from build123d import *

# Parameters (mm, degrees)
SKETCH1_R           = 13.5
BOSS_EXTRUDE1_DEPTH = 60
CUT_EXTRUDE1_START  = -30
SKETCH2_R           = 13.5
SKETCH2_R_2         = 12
CUT_EXTRUDE1_DEPTH  = 30
SKETCH3_R           = 2
BOSS_EXTRUDE2_DEPTH = 7
SKETCH4_W           = 23.8117618
SKETCH4_H           = 3
BOSS_EXTRUDE3_DEPTH = 2


with BuildPart() as part:
    # Sketch1 → Boss-Extrude1 (new body)
    with BuildSketch(Plane.XY):
        Circle(SKETCH1_R)
    extrude(amount=BOSS_EXTRUDE1_DEPTH)

    # Sketch2 → Cut-Extrude1 (cut)
    with BuildSketch(Plane.XY.offset(60).offset(CUT_EXTRUDE1_START)):
        Circle(SKETCH2_R)
        Circle(SKETCH2_R_2, mode=Mode.SUBTRACT)
    extrude(amount=CUT_EXTRUDE1_DEPTH, mode=Mode.SUBTRACT)

    # Sketch3 → Boss-Extrude2 (add)
    with BuildSketch(Plane(origin=(0, 0, 0), x_dir=(-1, 0, 0), z_dir=(0, 0, -1))):
        Circle(SKETCH3_R)
        with Locations(Location((-8, 0, 0), (0, 0, 180))):
            Circle(SKETCH3_R)
    extrude(amount=BOSS_EXTRUDE2_DEPTH)

    # Sketch4 → Boss-Extrude3 (add)
    with BuildSketch(Plane.XY.offset(60)):
        Rectangle(SKETCH4_W, SKETCH4_H)
    extrude(amount=BOSS_EXTRUDE3_DEPTH)


solid = part.part
CAD build for the part. Positions are in the model's coordinates, mm. A direction names the side the tool comes from. Coordinates: 2 decimals unless noted, no trailing zeros. Write each loop counter-clockwise with the first axis right and the second up, starting at its lowest first coordinate (ties: lowest second). Pieces come first, ordered by that corner, then holes. Notation, with made-up numbers: M 52,84 L 107,84 A28 ccw 107,107 Z; hole C 76.25,-4.5 d8. An arc over 180 degrees is marked long. Return JSON: item names as keys, results as strings.
Item 1: Drop flat-ended pins along their axis: pin 1 Ø1.5 at (x, y) = (6.5, 3) entering from +Z; pin 2 Ø1.6 at (y, z) = (-0.5, 61) entering from -X; pin 3 Ø5 at (x, z) = (-10.5, 49.5) entering from +Y. Give the stop position or say it passes through.
Findings below:
{"pin 1": "stops at z = 60", "pin 2": "stops at x = -11.91", "pin 3": "stops at y = 8.94"}
Item 2: Slice it at B-B, the plane x = 0. Write the cut outline in (y, z), and give its area (3 significant figures).
Findings below:
{"outline": "M -13.5,0 L -2,0 L -2,-7 L 2,-7 L 2,0 L 13.5,0 L 13.5,30 L 12,30 L 12,60 L 1.5,60 L 1.5,62 L -1.5,62 L -1.5,60 L -12,60 L -12,30 L -13.5,30 Z", "area": "1,560 mm2"}
Item 3: Two-plate mould, pull along X, no slides. Class faces 1 (the flat face through (11.906, 0, 61)), 2 (the flat face through (0, 6, 60)), 3 (the cylindrical face through (6, 0, -3)): +X half, -X half, draft (parallel to the pull), parting line (faces both ways), or undercut.
Findings below:
{"face 1": "+X half", "face 2": "draft", "face 3": "undercut"}
Item 4: Which spindle directions (+Z, -Z, +X, -X, +Y, -Y) get a long thin tool onto all of the face, cutting with end or side? Do faces 4 (the cylindrical face through (0, -2, -3)), 5 (the flat face through (0, -6, 60)), 6 (the flat face through (0, 1.5, 61)), 7 (the flat face through (-12, -2, 30)). Say none if no direction does.
Findings below:
{"face 4": "-Z", "face 5": "+Z, +X, -X, -Y", "face 6": "+Z, +X, -X, +Y", "face 7": "+Z"}
Item 5: Probe line 1 (Z direction, x = 3, y = 2.5); line 2 (Z direction, x = -2.5, y = 0.5); line 3 (Y direction, x = -1.5, z = 49.5). List the from-to ranges inside material, lowest first. Write a range as from..to.
Findings below:
{"line 1": "z = 0..60", "line 2": "z = 0..62", "line 3": "y = -11.91..11.91"}
Item 6: Slice it at C-C, the plane z = 53.5. Write the cut outline in (x, y), and give its area (3 significant figures).
Findings below:
{"outline": "C 0,0 d24", "area": "452 mm2"}
Item 7: Slice it at D-D, the plane x = 9.25. Write the cut outline in (y, z).
Findings below:
{"outline": "M -9.83,0 L -1.56,0 L -1.56,-7 L 1.56,-7 L 1.56,0 L 9.83,0 L 9.83,30 L 7.64,30 L 7.64,60 L 1.5,60 L 1.5,62 L -1.5,62 L -1.5,60 L -7.64,60 L -7.64,30 L -9.83,30 Z"}
Item 8: Slice it at A-A, the plane y = 0. Write the cut outline in (x, z), and give its area (3 significant figures).
Findings below:
{"outline": "M -13.5,0 L -2,0 L -2,-7 L 2,-7 L 2,0 L 6,0 L 6,-7 L 10,-7 L 10,0 L 13.5,0 L 13.5,30 L 12,30 L 12,60 L 11.91,60 L 11.91,62 L -11.91,62 L -11.91,60 L -12,60 L -12,30 L -13.5,30 Z", "area": "1,630 mm2"}
